```python
from build123d import *

# Parameters (mm, degrees)
F0_W     = 190.5
F0_H     = 38.1
F1_DEPTH = 12.7
F3_D     = 25.4


with BuildPart() as f1:
    # F0 (on Front) → F1 (new body)
    with BuildSketch(Plane.XZ):
        with Locations((6.291108, 6.421452)):
            Rectangle(F0_W, F0_H)
    extrude(amount=F1_DEPTH)

    # F3 (through all)
    with Locations(Plane.XZ.offset(12.7)):
        with Locations((-69.908892, 6.421452), (82.491108, 6.421452)):
            Hole(F3_D / 2)


solid = f1.part
```
Input: part model. Units: mm. Frame: model coordinates. Give positions to 0.01 mm unless a question says otherwise; leave off trailing zeros. Order: outer loops, then holes, each group sorted by start corner. A loop starts at its lowest first (then second) coordinate and runs counter-clockwise, first axis right, second up. Notation, with made-up numbers: M 40,36.25 L 50,36.25 A15 cw 50,60.25 Z; hole C 57,22.25 d8. An arc over 180 degrees is marked long. Return JSON: item names as keys, results as strings.
Item 1: Cut plane C-C (y = -8). Return loops of the section in (x, z), then the cut area to 3 significant figures.
Solutions:
{"outline": "M -88.96,-12.63 L 101.54,-12.63 L 101.54,25.47 L -88.96,25.47 Z; hole C -69.91,6.42 d25.4; hole C 82.49,6.42 d25.4", "area": "6,240 mm^2"}
Item 2: Cut plane A-A (z = 8.5). Return loops of the section in (x, y), then the cut area to 3 significant figures.
Solutions:
{"outline": "M -88.96,-12.7 L -82.44,-12.7 L -82.44,0 L -88.96,0 Z; M -57.38,-12.7 L 69.96,-12.7 L 69.96,0 L -57.38,0 Z; M 95.02,-12.7 L 101.54,-12.7 L 101.54,0 L 95.02,0 Z", "area": "1,780 mm^2"}
Item 3: Pull-direction query (Z, two-part tool) for faces 1 (the flat face through (101.541, -6, 6)), 2 (the cylindrical face through (95.18, -6.26, 6.98)), 3 (the flat face through (5, -6, 25.471)); classes: +Z half, -Z half, draft (parallel to the pull), parting line (faces both ways), or undercut.
Solutions:
{"face 1": "draft", "face 2": "undercut", "face 3": "+Z half"}
Item 4: Cut plane B-B (x = 80). Return loops of the section in (y, z), then the cut area to 3 significant figures.
Solutions:
{"outline": "M -12.7,-12.63 L 0,-12.63 L 0,-6.03 L -12.7,-6.03 Z; M -12.7,18.87 L 0,18.87 L 0,25.47 L -12.7,25.47 Z", "area": "168 mm^2"}
Item 5: Cut plane D-D (z = 0). Return loops of the section in (x, y), then the cut area to 3 significant figures.
Solutions:
{"outline": "M -88.96,-12.7 L -80.87,-12.7 L -80.87,0 L -88.96,0 Z; M -58.95,-12.7 L 71.53,-12.7 L 71.53,0 L -58.95,0 Z; M 93.45,-12.7 L 101.54,-12.7 L 101.54,0 L 93.45,0 Z", "area": "1,860 mm^2"}
Item 6: Ray query, probe 1 along X at (y, z) = (-1.25, 6.5); probe 2 along X at (y, z) = (-4.5, -4); probe 3 along Z at (x, y) = (82.5, -2.25). Return the intervals inside material, ascending.
Solutions:
{"probe 1": "-88.96 to -82.61, -57.21 to 69.79, 95.19 to 101.54", "probe 2": "-88.96 to -77.17, -62.65 to 75.23, 89.75 to 101.54", "probe 3": "-12.63 to -6.28, 19.12 to 25.47"}
